Design review of the part built by this model. Coordinates are the model's own, in mm. Face numbers are marked on the shaded views. A direction names the side the tool comes from. Coordinates: 2 decimals unless noted, no trailing zeros. Write each loop counter-clockwise with the first axis right and the second up, starting at its lowest first coordinate (ties: lowest second). Pieces come first, ordered by that corner, then holes. Notation, with made-up numbers: (-17.5, 39) - (29.5, 39) arc R31 cw to (29.5, 70) - close; hole circle Ø7 at (82, -39). An arc over 180 degrees is marked (long way). One line per item, written item: value.
from build123d import *

# Parameters (mm, degrees)
F1_DEPTH  = 3.25
F3_DEPTH  = 0.5
F5_DEPTH  = 0.5
F7_DEPTH  = 0.5
F9_DEPTH  = 0.5
F10_W     = 24
F10_H     = 2.8
F11_DEPTH = 20
F13_DEPTH = 1.4
F14_W     = 8
F14_H     = 1
F15_DEPTH = 25
F16_R     = 1


# Not quite as in the source:
# - ends of sketch curves that miss each other by under 0.0002 mm in the source are joined


with BuildPart() as f1:
    # F0 (on Front) → F1 (new body, symmetric)
    with BuildSketch(Plane.XZ):
        Polygon((18, 18), (0, 18), (-18, 18), (-35, 0), (0, -47), (35, 0), align=None)
    extrude(amount=F1_DEPTH, both=True)

    # F2 (on face) → F3 (cut)
    with BuildSketch(Plane.XZ.offset(3.25)):
        Polygon((15.8447675538, 13), (-15.8447675538, 13), (-28.4822773709, -0.3808927475), (1.162e-07, -38.628522516), (28.4822775009, -0.3808928851), align=None)
    extrude(amount=-F3_DEPTH, mode=Mode.SUBTRACT)

    # F4 (on face) → F5 (cut)
    with BuildSketch(Plane(origin=(0, 3.25, 0), x_dir=(-1, 0, 0), z_dir=(0, 1, 0))):
        Polygon((28.482277527, -0.3808925379), (15.8447676545, 13.0000002682), (-15.8447670441, 13.0000002682), (-28.4822772579, -0.3808928993), (0, -38.6285223599), align=None)
    extrude(amount=-F5_DEPTH, mode=Mode.SUBTRACT)

    # F6 (on face) → F7 (cut)
    with BuildSketch(Plane.XZ.offset(2.75)):
        Polygon((-15.8447675538, -17.3512630734), (-15.8447675538, 13), (-28.4822773709, -0.3808927475), align=None)
        Polygon((28.4822775009, -0.3808928851), (15.8447675538, 13), (15.8447675538, -17.3512633855), align=None)
        Polygon((0, -8.4544227059), (-11.8447675538, 6.5455772941), (-11.8447675538, -22.7226916448), (1.162e-07, -38.628522516), (11.8447675538, -22.7226919569), (11.8447675538, 6.5455772941), align=None)
        Polygon((11.8447675538, 13), (-11.8447675538, 13), (0, -2), align=None)
    extrude(amount=-F7_DEPTH, mode=Mode.SUBTRACT)

    # F8 (on face) → F9 (cut)
    with BuildSketch(Plane(origin=(0, 2.75, 0), x_dir=(-1, 0, 0), z_dir=(0, 1, 0))):
        Polygon((-15.8447675538, -17.3512633855), (-15.8447675538, 13), (-28.4822772579, -0.3808928993), align=None)
        Polygon((0, -8.4544227059), (-11.8447675538, 6.5455772941), (-11.8447675538, -22.7226919569), (0, -38.6285223599), (11.8447675538, -22.7226916448), (11.8447675538, 6.5455772941), align=None)
        Polygon((-11.8447675538, 13), (0, -2), (11.8447675538, 13), align=None)
        Polygon((28.482277527, -0.3808925379), (15.8447676545, 13.0000002682), (15.8447675538, -17.3512630734), align=None)
    extrude(amount=-F9_DEPTH, mode=Mode.SUBTRACT)

    # F10 (on face) → F11 (cut)
    with BuildSketch(Plane.XY.offset(18)):
        Rectangle(F10_W, F10_H)
    extrude(amount=-F11_DEPTH, mode=Mode.SUBTRACT)

    # F12 (on Front) → F13 (cut, symmetric)
    with BuildSketch(Plane.XZ):
        with BuildLine():
            Line((12, -2), (-12, -2))
            ThreePointArc((-12, -2), (0, -14), (12, -2))
        make_face()
    extrude(amount=F13_DEPTH, both=True, mode=Mode.SUBTRACT)

    # F14 (on face) → F15 (cut)
    with BuildSketch(Plane.XZ.offset(3.25)):
        with Locations((0, 15.5)):
            Rectangle(F14_W, F14_H)
    extrude(amount=-F15_DEPTH, mode=Mode.SUBTRACT)

    # F16
    f16_edges = [f1.edges().sort_by_distance(p)[0] for p in [
        (0, 0, -47),
        (35, 0, 0),
        (-35, 0, 0),
        (-18, 0, 18),
        (18, 0, 18),
    ]]
    fillet(f16_edges, radius=F16_R)


solid = f1.part
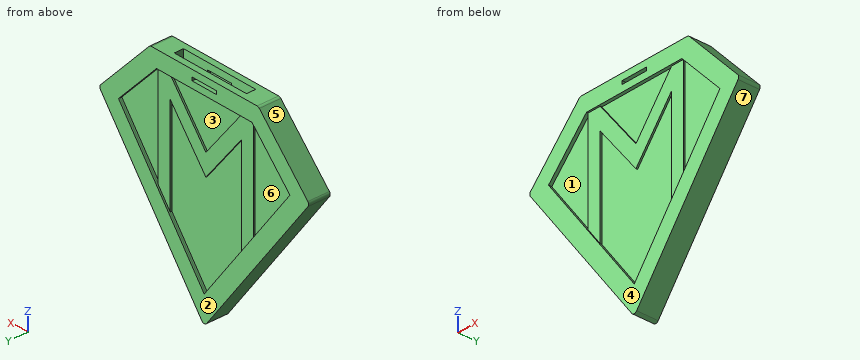
1. Mouldability with a two-part tool opening along Z and no side actions: class the marked faces 4, 5, 6 and 7 as released by +Z, released by -Z, zero draft, split by the parting line, or undercut.
Answer block:
face 4: zero draft
face 5: released by +Z
face 6: undercut
face 7: released by -Z
2. For the marked faces 1, 2 and 3, list the 3-axis set-ups (+Z, -Z, +X, -X, +Y, -Y) from which the entire face can be reached by the end or side of a thin tool; tool diameter is ignored.
Answer block:
face 1: -Y
face 2: +Z, -Z, +X, -X, +Y
face 3: +Y
3. Consider section C-C, the plane z = -23.5. Write out the cut boundary in (x, y).
Answer block:
outline: (-17.5, -3.25) - (-11.27, -3.25) - (-11.27, -2.25) - (11.27, -2.25) - (11.27, -3.25) - (17.5, -3.25) - (17.5, 3.25) - (11.27, 3.25) - (11.27, 2.25) - (-11.27, 2.25) - (-11.27, 3.25) - (-17.5, 3.25) - close
4. Insertion check: pin 1 Ø0.6 at (x, y) = (-1.5, -2.5) entering from -Z; pin 2 Ø1.1 at (y, z) = (-2.5, 15.5) entering from +X; pin 3 Ø1.1 at (y, z) = (-2, 15.5) entering from -X. Each pin has a flat end and moves straight along its axis. Give the tip position at first contact, or say it passes through.
Answer block:
pin 1: stops at z = -45.39
pin 2: stops at x = 20.88
pin 3: stops at x = -20.88
5. Wall thickness on line 1 along Y through (x, z) = (-0.5, 9.5); line 2 along X through (y, z) = (-1.25, 11); line 3 along Y through (x, z) = (-2, -21.5): over which ranges is each line inside the solid? List them lowest first.
Answer block:
line 1: y = -2.25 to -1.4, 1.4 to 2.25
line 2: x = -24.61 to -12, 12 to 24.61
line 3: y = -2.25 to 2.25
6. Consider section A-A, the plane z = -30. Write out the cut boundary in (x, y), then the cut area to 3 significant figures.
Answer block:
outline: (-12.66, -3.25) - (-6.43, -3.25) - (-6.43, -2.25) - (6.43, -2.25) - (6.43, -3.25) - (12.66, -3.25) - (12.66, 3.25) - (6.43, 3.25) - (6.43, 2.25) - (-6.43, 2.25) - (-6.43, 3.25) - (-12.66, 3.25) - close
area: 139 mm^2
7. Consider section B-B, the plane x = -13. Write out the cut boundary in (y, z), then the cut area to 3 significant figures.
Answer block:
outline: (-3.25, -29.54) - (3.25, -29.54) - (3.25, -21.17) - (2.75, -21.17) - (2.75, 13) - (3.25, 13) - (3.25, 18) - (-3.25, 18) - (-3.25, 13) - (-2.75, 13) - (-2.75, -21.17) - (-3.25, -21.17) - close
area: 275 mm^2
